```python
from build123d import *

# Parameters (mm, degrees)
F1_DEPTH = 20
F2_W     = 25
F2_H     = 12
F3_DEPTH = 12
F4_R     = 3
F5_DEPTH = 10
F6_R     = 3
F7_DEPTH = 10
F8_R     = 2.5
F9_DEPTH = 25


with BuildPart() as f1:
    # F0 (on Top) → F1 (new body)
    with BuildSketch(Plane.XY):
        Polygon((-9, 0), (0, 0), (9, 0), (9, 0.249999), (3.5, 5.749999), (0, 5.749999), (-3.5, 5.749999), (-9, 0.249999), align=None)
    extrude(amount=F1_DEPTH)

    # F2 (on Top) → F3 (join)
    with BuildSketch(Plane.XY):
        with Locations((0, 1.5)):
            Rectangle(F2_W, F2_H)
    extrude(amount=-F3_DEPTH)

    # F4 (on face) → F5 (cut)
    with BuildSketch(Plane.YZ.offset(12.5)):
        with Locations((1.5, -6)):
            Circle(F4_R)
    extrude(amount=-F5_DEPTH, mode=Mode.SUBTRACT)

    # F6 (on face) → F7 (cut)
    with BuildSketch(Plane(origin=(-12.5, 0, 0), x_dir=(0, -1, 0), z_dir=(-1, 0, 0))):
        with Locations((-1.5, -6)):
            Circle(F6_R)
    extrude(amount=-F7_DEPTH, mode=Mode.SUBTRACT)

    # F8 (on face) → F9 (cut)
    with BuildSketch(Plane.XZ):
        with Locations((0, 10)):
            Circle(F8_R)
    extrude(amount=-F9_DEPTH, mode=Mode.SUBTRACT)


solid = f1.part
```
Part model, mm, in its own coordinate system. A direction names the side the tool comes from. Round coordinates to 2 decimals unless told otherwise and drop trailing zeros. Loops run counter-clockwise (first coordinate to the right, second up) from the corner with the lowest first, then second, coordinate; pieces in that order, holes last. Notation, with made-up numbers: (-39, 24) -> (-31, 24) arc R22 ccw to (-31, 60) -> close; hole circle Ø4 at (-12, -16). An arc over 180 degrees is marked (long way). Use a Markdown table: item, result.
1) Cut at A-A, the plane x = 0. List the corners of the cut face in (y, z).
The answers:
| item | result |
|---|---|
| outline | (-4.5, -12) -> (7.5, -12) -> (7.5, 0) -> (5.75, 0) -> (5.75, 7.5) -> (0, 7.5) -> (0, 0) -> (-4.5, 0) -> close; (0, 12.5) -> (5.75, 12.5) -> (5.75, 20) -> (0, 20) -> close |
2) Pull direction Y, two halves, no side cores. Call faces 1 (the cylindrical face through (7.57, 1.109, -3.026)), 2 (the flat face through (-6.21, 3.04, 9.86)), 3 (the flat face through (0, 2, -12)): pulls with the +Y half, pulls with the -Y half, needs draft (parallel to the pull), parting line crosses it, or undercut.
The answers:
| item | result |
|---|---|
| face 1 | undercut |
| face 2 | pulls with the +Y half |
| face 3 | needs draft |
3) Tool access for faces 4 (the cylindrical face through (-7.57, 1.891, -3.026)), 5 (the flat face through (2.5, 1, -6)), 6 (the flat face through (2, 5.75, 8)): list every direction of +Z, -Z, +X, -X, +Y, -Y with a clear straight run to the whole face (end or side of a thin tool).
The answers:
| item | result |
|---|---|
| face 4 | -X |
| face 5 | +X |
| face 6 | +Z, +X, -X, +Y |
4) Probe line 1 (Z direction, x = -6.25, y = 1.5); line 2 (Z direction, x = 8.75, y = 1.5); line 3 (Z direction, x = -5, y = -2.25). List the from-to ranges inside material, lowest first. Write a range as [from, to].
The answers:
| item | result |
|---|---|
| line 1 | z = [-12, -9], [-3, 20] |
| line 2 | z = [-12, -9], [-3, 0] |
| line 3 | z = [-12, 0] |
5) Cut at C-C, the plane y = 1.5. List the corners of the cut face in (x, z).
The answers:
| item | result |
|---|---|
| outline | (-12.5, -12) -> (12.5, -12) -> (12.5, -9) -> (2.5, -9) -> (2.5, -3) -> (12.5, -3) -> (12.5, 0) -> (7.75, 0) -> (7.75, 20) -> (-7.75, 20) -> (-7.75, 0) -> (-12.5, 0) -> (-12.5, -3) -> (-2.5, -3) -> (-2.5, -9) -> (-12.5, -9) -> close; hole circle Ø5 at (0, 10) |
6) Cut at B-B, the plane z = 10. List the corners of the cut face in (x, y), and give its area (3 significant figures).
The answers:
| item | result |
|---|---|
| outline | (-9, 0) -> (-2.5, 0) -> (-2.5, 5.75) -> (-3.5, 5.75) -> (-9, 0.25) -> close; (2.5, 0) -> (9, 0) -> (9, 0.25) -> (3.5, 5.75) -> (2.5, 5.75) -> close |
| area | 44.5 mm2 |
7) Drop flat-ended pins along their axis: pin 1 Ø7.5 at (x, z) = (-0.5, 12) entering from +Y; pin 2 Ø1.8 at (y, z) = (1, -5.5) entering from -X; pin 3 Ø2 at (y, z) = (3, -8) entering from +X; pin 4 Ø3 at (y, z) = (1, 11) entering from +X. Give the stop position or say it passes through.
The answers:
| item | result |
|---|---|
| pin 1 | stops at y = 5.75 |
| pin 2 | stops at x = -2.5 |
| pin 3 | stops at x = 12.5 |
| pin 4 | stops at x = 9 |
8) Cut at D-D, the plane x = 4.75. List the corners of the cut face in (y, z), and give its area (3 significant figures).
The answers:
| item | result |
|---|---|
| outline | (-4.5, -12) -> (7.5, -12) -> (7.5, 0) -> (4.5, 0) -> (4.5, 20) -> (0, 20) -> (0, 0) -> (-4.5, 0) -> close; hole circle Ø6 at (1.5, -6) |
| area | 206 mm2 |
